Verification items for the finished model (mm, model axes). Face numbers are marked on the shaded views. Give positions to 0.01 mm unless a question says otherwise; leave off trailing zeros. Write each loop counter-clockwise with the first axis right and the second up, starting at its lowest first coordinate (ties: lowest second). Pieces come first, ordered by that corner, then holes. Notation, with made-up numbers: (-34, -36.5) - (-30, -36.5) arc R7 ccw to (-30, -27.5) - close; hole circle Ø9 at (16.25, -34.5). An arc over 180 degrees is marked (long way). Answer as a JSON object with one key per item and string values. Group by question number.
Item 1: Scan lines: line 1 along Y through (x, z) = (15, -2); line 2 along X through (y, z) = (38.5, 2.5); line 3 along Y through (x, z) = (-1, 2.5). Record each from-to range of solid material in increasing order. Write a range as [from, to].
Item 2: Sectioned sample at A-A, the plane x = -15. Record the boundary of the cut face in (y, z).
Item 3: Go/stop test with flat-tipped pins: pin 1 (4 mm diameter, centred on x = -1, y = -4.5, fed in from +Z); pin 2 (3 mm diameter, centred on x = 0, y = -3, fed in from +Z). Record where each tip stops, or that it passes through.
Item 4: Draft check along Y on the marked faces 1, 2 and 3. Enter one of: +Y half, -Y half, draft (parallel to the pull), parting line (faces both ways), or undercut.
Item 5: Sectioned sample at B-B, the plane y = 0. Record the boundary of the cut face in (x, z), and give its area (3 significant figures).
Item 6: Sectioned sample at C-C, the plane x = 22. Record the boundary of the cut face in (y, z), and give its area (3 significant figures).
```python
from build123d import *

# Parameters (mm, degrees)
SKETCH_1_W      = 50
SKETCH_1_H      = 80
SKETCH_1_R      = 4.1
SKETCH_1_R_2    = 2.1
EXTRUDE_1_DEPTH = 3
CHAMFER_2_SIZE  = 4
CHAMFER_3_SIZE  = 2


with BuildPart() as part:
    # 草图1 → 凸台-拉伸1 (new, symmetric)
    with BuildSketch(Plane.XY):
        with Locations((0, 10)):
            Rectangle(SKETCH_1_W, SKETCH_1_H)
        Circle(SKETCH_1_R, mode=Mode.SUBTRACT)
        with Locations((-15, 40)):
            Circle(SKETCH_1_R_2, mode=Mode.SUBTRACT)
        with Locations((15, 40)):
            Circle(SKETCH_1_R_2, mode=Mode.SUBTRACT)
    extrude(amount=EXTRUDE_1_DEPTH, both=True)

    # 倒角2
    chamfer_2_edges = [part.edges().sort_by_distance(p)[0] for p in [
        (-4.1, 0, 3),
        (-25, 50, 0),
        (25, 50, 0),
        (25, -30, 0),
        (-25, -30, 0),
    ]]
    chamfer(chamfer_2_edges, length=CHAMFER_2_SIZE)

    # 倒角3
    chamfer_3_edges = [part.edges().sort_by_distance(p)[0] for p in [
        (-17.1, 40, 3),
        (12.9, 40, 3),
    ]]
    chamfer(chamfer_3_edges, length=CHAMFER_3_SIZE)


solid = part.part
```
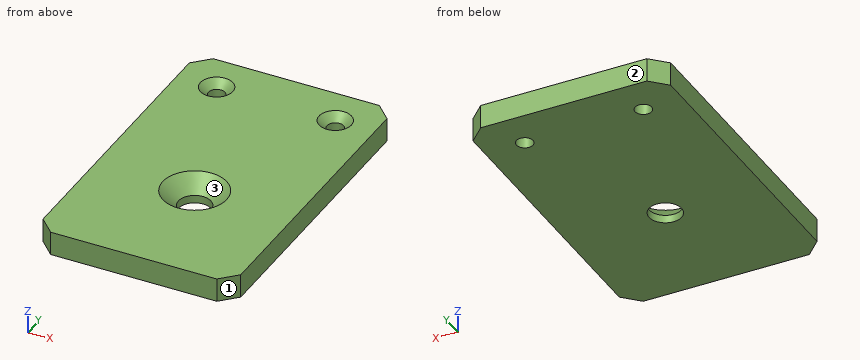
Geometry check:
{
 "1": {"line 1": "[-30, 37.9], [42.1, 50]", "line 2": "[-25, -18.27], [-11.73, 11.73], [18.27, 25]", "line 3": "[-30, -7.53], [7.53, 50]"},
 "2": {"outline": "(-30, -3) - (37.9, -3) - (37.9, 1) - (35.9, 3) - (-30, 3) - close; (42.1, -3) - (50, -3) - (50, 3) - (44.1, 3) - (42.1, 1) - close"},
 "3": {"pin 1": "z = 1.51", "pin 2": "z = -0.6"},
 "4": {"face 1": "-Y half", "face 2": "+Y half", "face 3": "undercut"},
 "5": {"outline": "(-25, -3) - (-4.1, -3) - (-4.1, -1) - (-8.1, 3) - (-25, 3) - close; (4.1, -3) - (25, -3) - (25, 3) - (8.1, 3) - (4.1, -1) - close", "area": "235 mm^2"},
 "6": {"outline": "(-29, -3) - (49, -3) - (49, 3) - (-29, 3) - close", "area": "468 mm^2"}
}
